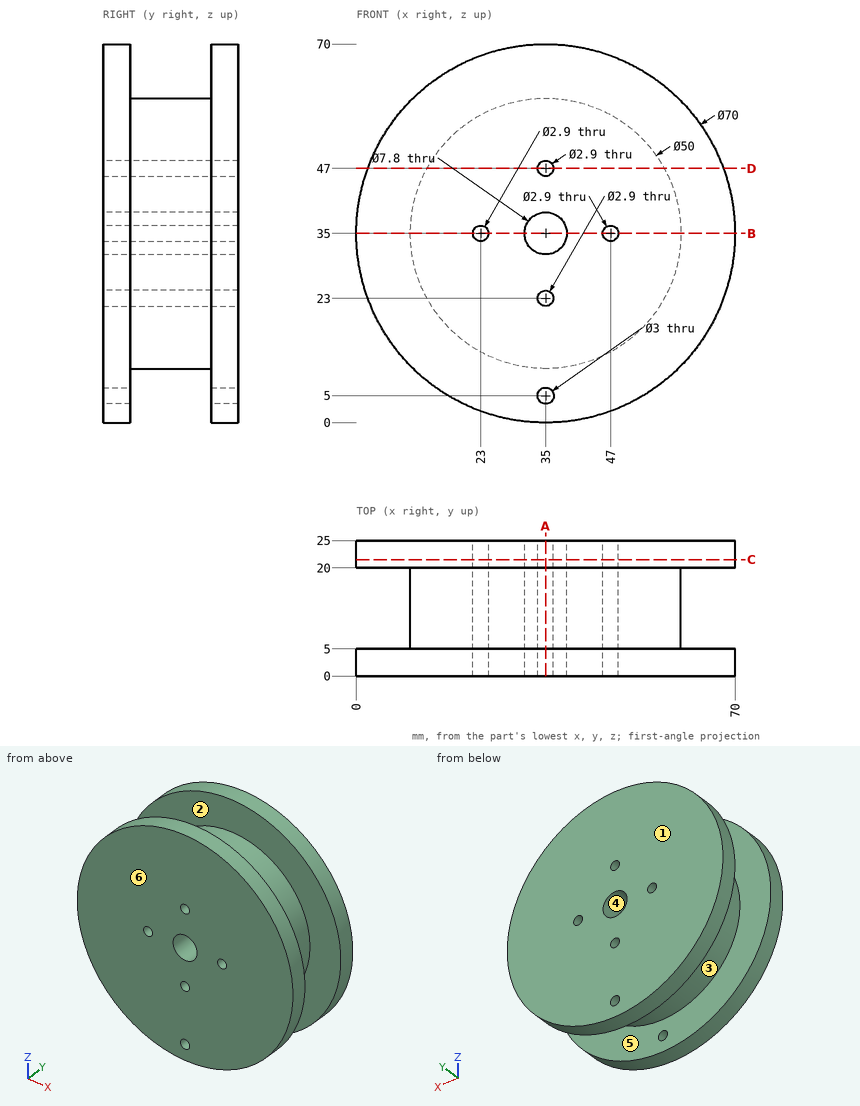
Source: three-view drawing plus pictorial views. Frame: mm from the lowest corner of the part. A direction names the side the tool comes from. Round coordinates to 2 decimals unless told otherwise and drop trailing zeros. Order: outer loops, then holes, each group sorted by start corner. A loop starts at its lowest first (then second) coordinate and runs counter-clockwise, first axis right, second up. Notation, with made-up numbers: (62, 42.25) - (72, 42.25) arc R19 cw to (72, 75.25) - close; hole circle Ø6 at (-39, 46.25). An arc over 180 degrees is marked (long way). Answer in a Markdown table with one row per item.
Item 1: Section query A-A (x = 35). Give the number of separate pieces and of enclosed holes in the cut face, then the cut area to 3 significant figures.
Model answer:
| item | result |
|---|---|
| separate pieces | 6 |
| enclosed holes | 0 |
| area | 1,080 mm² |
Item 2: Section query D-D (z = 47). Return the cut outline in (x, y), then the cut area to 3 significant figures.
Model answer:
| item | result |
|---|---|
| outline | (2.12, 0) - (33.55, 0) - (33.55, 25) - (2.12, 25) - (2.12, 20) - (13.07, 20) - (13.07, 5) - (2.12, 5) - close; (36.45, 0) - (67.88, 0) - (67.88, 5) - (56.93, 5) - (56.93, 20) - (67.88, 20) - (67.88, 25) - (36.45, 25) - close |
| area | 1,240 mm² |
Item 3: Pin query (flat end, axial travel): pin 1 (1.5 mm diameter, centred on x = 23, y = 3.5, fed in from -Z); pin 2 (5 mm diameter, centred on x = 15.5, y = 8, fed in from -Z); pin 3 (1.5 mm diameter, centred on x = 34, y = 11, fed in from +Z). Return the tip coordinate at first contact, or that it passes through.
Model answer:
| item | result |
|---|---|
| pin 1 | stops at z = 1.86 |
| pin 2 | stops at z = 16.67 |
| pin 3 | stops at z = 60 |
Item 4: Mould query, pull axis Y, two halves, no side actions, for the marked faces 3, 4, 5 and 6. Classes: released by +Y, released by -Y, zero draft, split by the parting line, or undercut.
Model answer:
| item | result |
|---|---|
| face 3 | undercut |
| face 4 | zero draft |
| face 5 | undercut |
| face 6 | released by -Y |
Item 5: Section query C-C (y = 21.5). Return the cut outline in (x, z), then the cut area to 3 significant figures.
Model answer:
| item | result |
|---|---|
| outline | circle Ø70 at (35, 35); hole circle Ø2.9 at (23, 35); hole circle Ø7.8 at (35, 35); hole circle Ø3 at (35, 5); hole circle Ø2.9 at (35, 23); hole circle Ø2.9 at (35, 47); hole circle Ø2.9 at (47, 35) |
| area | 3,770 mm² |
Item 6: Reachability of the marked faces 1 and 2 from +Z, -Z, +X, -X, +Y, -Y: full face, straight path, thin tool, end or side. Return the list, or none.
Model answer:
| item | result |
|---|---|
| face 1 | +Z, -Z, +X, -X, +Y |
| face 2 | none |
Item 7: Line query: line 1 (X direction, y = 10.5, z = 35); line 2 (Y direction, x = 36, z = 60.5); line 3 (Z direction, x = 34, y = 6). Output: solid intervals per line, ascending.
Model answer:
| item | result |
|---|---|
| line 1 | x = 10 to 21.55, 24.45 to 31.1, 38.9 to 45.55, 48.45 to 60 |
| line 2 | y = 0 to 5, 20 to 25 |
| line 3 | z = 10.02 to 21.95, 24.05 to 31.23, 38.77 to 45.95, 48.05 to 59.98 |
Item 8: Section query B-B (z = 35). Return the cut outline in (x, y), then the cut area to 3 significant figures.
Model answer:
| item | result |
|---|---|
| outline | (0, 0) - (21.55, 0) - (21.55, 25) - (0, 25) - (0, 20) - (10, 20) - (10, 5) - (0, 5) - close; (24.45, 0) - (31.1, 0) - (31.1, 25) - (24.45, 25) - close; (38.9, 0) - (45.55, 0) - (45.55, 25) - (38.9, 25) - close; (48.45, 0) - (70, 0) - (70, 5) - (60, 5) - (60, 20) - (70, 20) - (70, 25) - (48.45, 25) - close |
| area | 1,110 mm² |
